Part model, mm, in its own coordinate system. Face numbers are marked on the shaded views. A direction names the side the tool comes from. Coordinates: 2 decimals unless noted, no trailing zeros. Write each loop counter-clockwise with the first axis right and the second up, starting at its lowest first coordinate (ties: lowest second). Pieces come first, ordered by that corner, then holes. Notation, with made-up numbers: (-11.5, 58.5) - (-2.5, 58.5) arc R20 cw to (-2.5, 65.5) - close; hole circle Ø1 at (19, 14.5). An arc over 180 degrees is marked (long way). Write each question's results on one line, items separated by ' | '.
from build123d import *

# Parameters (mm, degrees)
SKETCH_1_W          = 10
SKETCH_1_H          = 20
SKETCH_1_W_2        = 8
SKETCH_1_H_2        = 18
EXTRUDE_1_DEPTH     = 40
SKETCH_2_R          = 2
CUT_EXTRUDE_1_DEPTH = 43.426406871
SKETCH_3_R          = 2
CUT_EXTRUDE_2_DEPTH = 46


with BuildPart() as part:
    # ｽｹｯﾁ1 → 押し出し-薄板1 (new body)
    with BuildSketch(Plane.XY):
        Rectangle(SKETCH_1_W, SKETCH_1_H)
        Rectangle(SKETCH_1_W_2, SKETCH_1_H_2, mode=Mode.SUBTRACT)
    extrude(amount=EXTRUDE_1_DEPTH)

    # ｽｹｯﾁ2 → ｶｯﾄ - 押し出し1 (cut, through all)
    with BuildSketch(Plane.ZY.offset(5)):
        with Locations((10, 0)):
            Circle(SKETCH_2_R)
        with Locations((30, 0)):
            Circle(SKETCH_2_R)
    extrude(amount=-CUT_EXTRUDE_1_DEPTH, mode=Mode.SUBTRACT)

    # ｽｹｯﾁ3 → ｶｯﾄ - 押し出し2 (cut, through all)
    with BuildSketch(Plane(origin=(0, 10, 0), x_dir=(1, 0, 0), z_dir=(0, 1, 0))):
        with Locations(Location((0, -5, 0), (0, 0, 270))):
            Circle(SKETCH_3_R)
        with Locations(Location((0, -35, 0), (0, 0, 90))):
            Circle(SKETCH_3_R)
    extrude(amount=-CUT_EXTRUDE_2_DEPTH, mode=Mode.SUBTRACT)


solid = part.part
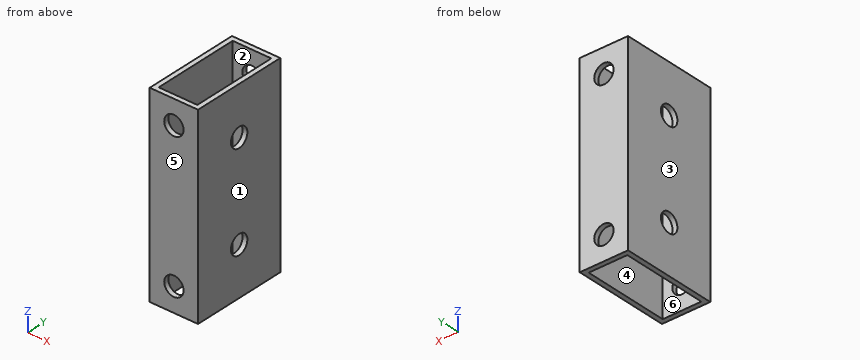
(1) Saw through at A-A on z = 10. Write the cut outline in (x, y).
Return value:
outline: (-5, -10) - (5, -10) - (5, -2) - (4, -2) - (4, -9) - (-4, -9) - (-4, -2) - (-5, -2) - close; (-5, 2) - (-4, 2) - (-4, 9) - (4, 9) - (4, 2) - (5, 2) - (5, 10) - (-5, 10) - close
(2) Flat gauge pin, fed straight in: P1, Ø2.5, axis at x = 0, z = 35, coming from the +Y side. Where does the tip first touch, or does it go through?
Return value:
P1: passes through
(3) 3-axis set-ups, long thin cutter, end or side, ignore diameter. For the marked faces 1 and 2: which of +Z, -Z, +X, -X, +Y, -Y reach the whole face in a straight line?
Return value:
face 1: +Z, -Z, +X, +Y, -Y | face 2: +Z, -Z
(4) Saw through at C-C on y = 0. Write the cut outline in (x, z), then the cut area to 3 significant figures.
Return value:
outline: (-5, 0) - (-4, 0) - (-4, 8) - (-5, 8) - close; (-5, 12) - (-4, 12) - (-4, 28) - (-5, 28) - close; (-5, 32) - (-4, 32) - (-4, 40) - (-5, 40) - close; (4, 0) - (5, 0) - (5, 8) - (4, 8) - close; (4, 12) - (5, 12) - (5, 28) - (4, 28) - close; (4, 32) - (5, 32) - (5, 40) - (4, 40) - close | area: 64.0 mm^2
(5) Saw through at B-B on x = 3. Write the cut outline in (y, z), then the cut area to 3 significant figures.
Return value:
outline: (-10, 0) - (-9, 0) - (-9, 40) - (-10, 40) - close; (9, 0) - (10, 0) - (10, 40) - (9, 40) - close | area: 80.0 mm^2
(6) Wall check: line 1 (X direction, y = 8.5, z = 4.5); line 2 (Y direction, x = 3.5, z = 23); line 3 (Y direction, x = -4.75, z = 10). Give the ranges that are in metal, low to high. Write a range as from..to.
Return value:
line 1: x = -5..-4, 4..5 | line 2: y = -10..-9, 9..10 | line 3: y = -10..-2, 2..10
(7) Saw through at D-D on y = -7. Write the cut outline in (x, z).
Return value:
outline: (-5, 0) - (-4, 0) - (-4, 40) - (-5, 40) - close; (4, 0) - (5, 0) - (5, 40) - (4, 40) - close
(8) Two-plate mould, pull along X, no slides. Class the marked faces 3, 4, 5 and 6: released by +X, released by -X, zero draft, split by the parting line, or undercut.
Return value:
face 3: released by -X | face 4: undercut | face 5: zero draft | face 6: undercut
